```python
from build123d import *

# Parameters (mm, degrees)
ESQUISSE1_W         = 30
ESQUISSE1_H         = 20
BOSS_EXTRU_1_DEPTH  = 30
SKETCH1_R           = 5
BOSS_EXTRUDE1_DEPTH = 10


with BuildPart() as part:
    # Esquisse1 → Boss.-Extru.1 (new body)
    with BuildSketch(Plane.XY):
        with Locations((-15, 10)):
            Rectangle(ESQUISSE1_W, ESQUISSE1_H)
    extrude(amount=BOSS_EXTRU_1_DEPTH)

    # Sketch1 → Boss-Extrude1 (add)
    with BuildSketch(Plane(origin=(0, 0, 0), x_dir=(1, 0, 0), z_dir=(0, 1, 0))):
        with Locations(Location((-20, -10, 0), (0, 0, 270))):
            Circle(SKETCH1_R)
    extrude(amount=-BOSS_EXTRUDE1_DEPTH)


solid = part.part
```
Geometry check sheet. Reference: the model listing, model coordinates, mm. A direction names the side the tool comes from. Coordinates: 2 decimals unless noted, no trailing zeros. Write each loop counter-clockwise with the first axis right and the second up, starting at its lowest first coordinate (ties: lowest second). Pieces come first, ordered by that corner, then holes. Notation, with made-up numbers: M 89,47.25 L 147,47.25 A23 ccw 147,58.25 Z; hole C 80,-8 d10. An arc over 180 degrees is marked long. Use one line per item in the form item = value. Start each with the question number.
1) Thickness scan on probe 1 along Y at (x, z) = (-7.75, 10); probe 2 along Z at (x, y) = (-17.25, -7.5); probe 3 along X at (y, z) = (-5.25, 10.75). Record the ranges inside material, lowest first. Write a range as from..to.
2) Go/stop test with flat-tipped pins: pin 1 Ø9 at (x, z) = (-12, 13.5) entering from -Y; pin 2 Ø1.5 at (y, z) = (-2.5, 12) entering from +X; pin 3 Ø5 at (y, z) = (-4.5, 26.5) entering from -X. Record where each tip stops, or that it passes through.
3) Section check B-B on x = -20. Enter the section's corners in (y, z), and give its area (3 significant figures).
4) Section check C-C on y = -0.75. Enter the section's corners in (x, z).
5) Section check D-D on z = 18.75. Enter the section's corners in (x, y), and give its area (3 significant figures).
6) Section check A-A on z = 13. Enter the section's corners in (x, y).
7) Set-up check for faces 1 (the cylindrical face through (-24.436, -4.93, 12.307)), 2 (the flat face through (-15, 10, 0)): record each of +Z, -Z, +X, -X, +Y, -Y from which the full face is reachable in a straight line by a thin tool's end or side.
Responses:
q1.probe_1 = 0..20
q1.probe_2 = 5.82..14.18
q1.probe_3 = -24.94..-15.06
q2.pin_1 = -10
q2.pin_2 = -15.16
q2.pin_3 = through
q3.outline = M -10,5 L 0,5 L 0,0 L 20,0 L 20,30 L 0,30 L 0,15 L -10,15 Z
q3.area = 700 mm2
q4.outline = C -20,10 d10
q5.outline = M -30,0 L 0,0 L 0,20 L -30,20 Z
q5.area = 600 mm2
q6.outline = M -30,0 L -24,0 L -24,-10 L -16,-10 L -16,0 L 0,0 L 0,20 L -30,20 Z
q7.face_1 = -Y
q7.face_2 = -Z, +X, -X, +Y, -Y
